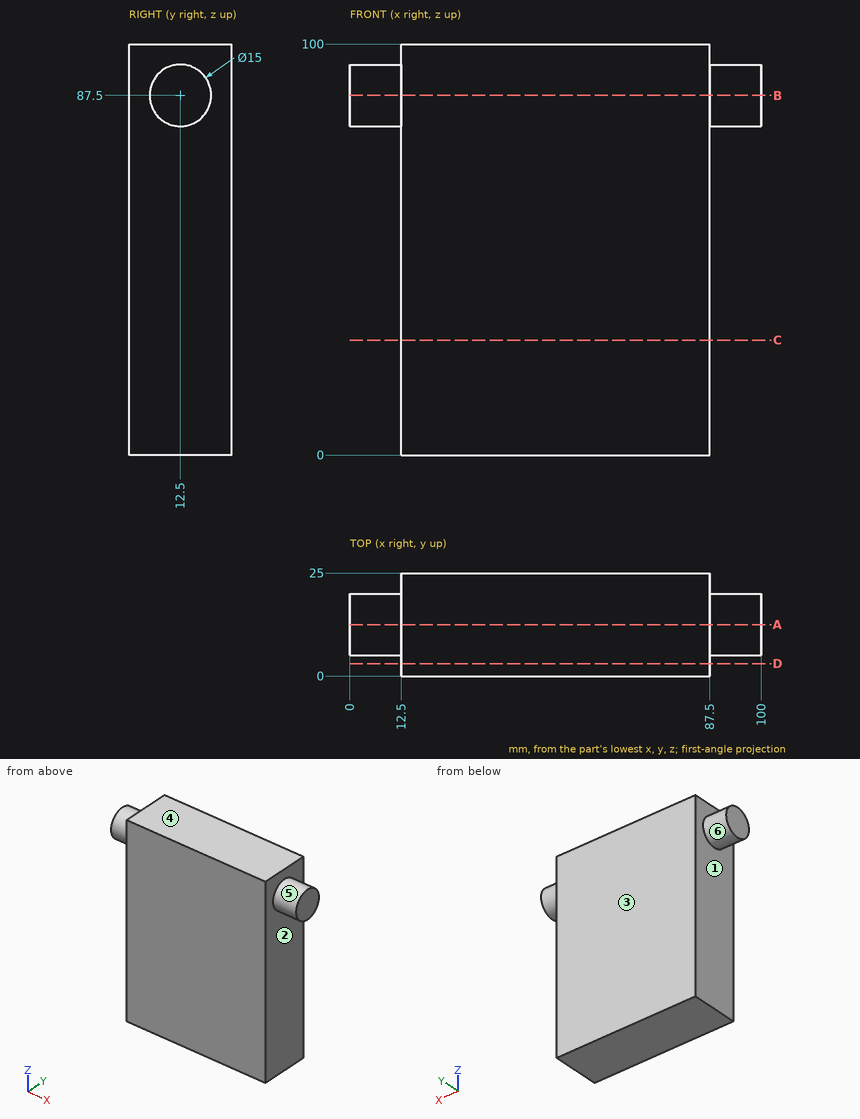
The figure shows three views and two pictorial views of one solid part (mm, origin at its lowest corner). Answer the questions. A direction names the side the tool comes from. Round coordinates to 2 decimals unless told otherwise and drop trailing zeros. Write each loop counter-clockwise with the first axis right and the second up, starting at its lowest first coordinate (ties: lowest second). Pieces come first, ordered by that corner, then holes. Notation, with made-up numbers: M 48,77.5 L 94,77.5 A21 cw 94,105.5 Z; hole C -11,-22.5 d3. An arc over 180 degrees is marked long. Use a Markdown table: item, result.
1) The part is cut by section C-C on z = 28. Give the vertices of the cut face in (x, y), plus the area to 4 significant figures.
Taken from the geometry:
| item | result |
|---|---|
| outline | M 12.5,0 L 87.5,0 L 87.5,25 L 12.5,25 Z |
| area | 1,875 mm2 |
2) The part is cut by section D-D on y = 3. Give the vertices of the cut face in (x, z), plus the area to 3 significant figures.
Taken from the geometry:
| item | result |
|---|---|
| outline | M 12.5,0 L 87.5,0 L 87.5,100 L 12.5,100 Z |
| area | 7,500 mm2 |
3) The part is cut by section B-B on z = 87.5. Give the vertices of the cut face in (x, y), plus the area to 3 significant figures.
Taken from the geometry:
| item | result |
|---|---|
| outline | M 0,5 L 12.5,5 L 12.5,0 L 87.5,0 L 87.5,5 L 100,5 L 100,20 L 87.5,20 L 87.5,25 L 12.5,25 L 12.5,20 L 0,20 Z |
| area | 2,250 mm2 |
4) Consider line 1 (X direction, y = 8.5, z = 55.5); line 2 (Y direction, x = 96.5, z = 91); line 3 (Y direction, x = 92, z = 86). Determine where each line is inside the solid, lowest interval first. Write a range as [from, to].
Taken from the geometry:
| item | result |
|---|---|
| line 1 | x = [12.5, 87.5] |
| line 2 | y = [5.87, 19.13] |
| line 3 | y = [5.15, 19.85] |
5) Determine the mould class of the marked faces 1, 2 and 3 for opening direction X: pulls with the +X half, pulls with the -X half, needs draft (parallel to the pull), parting line crosses it, or undercut.
Taken from the geometry:
| item | result |
|---|---|
| face 1 | pulls with the -X half |
| face 2 | pulls with the +X half |
| face 3 | needs draft |
6) Which of the six approach directions +Z, -Z, +X, -X, +Y, -Y give full straight-line access (tool end or side, diameter ignored) to the marked faces 4, 5 and 6?
Taken from the geometry:
| item | result |
|---|---|
| face 4 | +Z, +X, -X, +Y, -Y |
| face 5 | +X |
| face 6 | -X |
7) Flat-ended cylindrical pins translate along their axes: pin 1 (2 mm diameter, centred on y = 8.5, z = 15, fed in from -X); pin 2 (12.5 mm diameter, centred on y = 15.5, z = 66, fed in from +X). Find the tip coordinate at first contact, or state that the pin passes through.
Taken from the geometry:
| item | result |
|---|---|
| pin 1 | stops at x = 12.5 |
| pin 2 | stops at x = 87.5 |
8) The part is cut by section A-A on y = 12.5. Give the vertices of the cut face in (x, z), plus the area to 4 significant figures.
Taken from the geometry:
| item | result |
|---|---|
| outline | M 0,80 L 12.5,80 L 12.5,0 L 87.5,0 L 87.5,80 L 100,80 L 100,95 L 87.5,95 L 87.5,100 L 12.5,100 L 12.5,95 L 0,95 Z |
| area | 7,875 mm2 |
